from build123d import *

# Parameters (mm, degrees)
SKETCH1_W                 = 63.398443118
SKETCH1_H                 = 25.4
BOSS_EXTRUDE1_DEPTH       = 6.35
SKETCH2_W                 = 38.1
SKETCH2_H                 = 25.4
BOSS_EXTRUDE2_DEPTH       = 6.35
CUT_EXTRUDE3_DEPTH        = 60.875617776
TAP_DRILL_FOR_6_32_TAP1_D = 2.7051
F_1_4_CLEARANCE_HOLE1_D   = 6.7564


with BuildPart() as part:
    # Sketch1 → Boss-Extrude1 (new body)
    with BuildSketch(Plane.XY):
        with Locations((22.148778441, 406.4)):
            Rectangle(SKETCH1_W, SKETCH1_H)
    extrude(amount=BOSS_EXTRUDE1_DEPTH)

    # Sketch2 → Boss-Extrude2 (add)
    with BuildSketch(Plane(origin=(0, 0, 0), x_dir=(-1, 0, 0), z_dir=(0, 0, -1))):
        with Locations((-34.798, 406.4)):
            Rectangle(SKETCH2_W, SKETCH2_H)
    extrude(amount=BOSS_EXTRUDE2_DEPTH)

    # Sketch7 → Cut-Extrude3 (cut, through all)
    with BuildSketch(Plane(origin=(0, 419.1, 0), x_dir=(1, 0, 0), z_dir=(0, 1, 0))):
        with BuildLine():
            Line((-9.550443118, -0.242852773), (15.748, -0.242852773))
            ThreePointArc((15.748, -0.242852773), (15.919722843, -0.171722843), (15.990852773, 0))
            Line((15.990852773, 0), (15.990852773, 6.35))
            Line((15.990852773, 6.35), (15.748, 6.35))
            Line((15.748, 6.35), (15.748, 0))
            Line((15.748, 0), (-9.550443118, 0))
            Line((-9.550443118, 0), (-9.550443118, -0.242852773))
        make_face()
    extrude(amount=-CUT_EXTRUDE3_DEPTH, mode=Mode.SUBTRACT)

    # Tap Drill for #6-32 Tap1 (through all)
    with Locations(Plane.XY.offset(6.35)):
        with Locations((47.498, 406.4), (30.0355, 406.4)):
            Hole(TAP_DRILL_FOR_6_32_TAP1_D / 2)

    # 1/4 Clearance Hole1 (through all)
    with Locations(Plane.XY.offset(6.35)):
        with Locations((3.149556882, 406.4)):
            Hole(F_1_4_CLEARANCE_HOLE1_D / 2)


solid = part.part
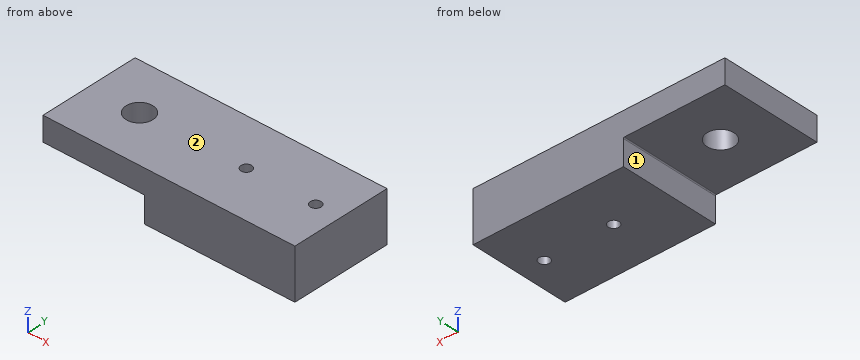
Can you work these out from the model? Positions are in its coordinate system, mm. Face numbers are marked on the shaded views. A direction names the side the tool comes from. Round coordinates to 2 decimals unless told otherwise and drop trailing zeros. Loops run counter-clockwise (first coordinate to the right, second up) from the corner with the lowest first, then second, coordinate; pieces in that order, holes last. Notation, with made-up numbers: (48, 54) - (98, 54) arc R33 ccw to (98, 88) - close; hole circle Ø3 at (74.5, 36). An arc over 180 degrees is marked (long way). Write item = value, one per line. Start each with the question number.
(1) If we section it at C-C (y = 413): Please give me the cut outline in (x, z).
(2) If I drill on probe 1 along X at (y, z) = (406.4, 2.75); probe 2 along X at (y, z) = (406.4, -0.75); probe 3 along Z at (x, y) = (-2.5, 395.75), over which ranges is the centre line in solid material (lowest first)? Write a range as [from, to].
(3) If we section it at A-A (z = 4.25): Please give me the cut outline in (x, y), and give its area (3 significant figures).
(4) For the marked faces 1 and 2, which set-ups out of +Z, -Z, +X, -X, +Y, -Y let a thin tool reach every point of the face, with its end or its side?
(5) For P1, Ø1.9, axis at y = 403.5, z = -1.5, coming from the -X side; P2, Ø12.5, axis at x = 7, y = 404.5, coming from the -Z side, each with a flat end and sliding along its axis, tell me the tip position at first contact or that it passes through.
(6) If we section it at B-B (y = 406.4): Please give me the cut outline in (x, z).
(7) If we section it at D-D (x = 1.5): Please give me the cut outline in (y, z).
Ans:
q1.outline = (-9.55, 0.24) - (15.75, 0.24) arc R0.24 cw to (15.99, 0) - (15.99, -6.35) - (53.85, -6.35) - (53.85, 6.35) - (-9.55, 6.35) - close
q2.probe_1 = [-9.55, -0.23], [6.53, 28.68], [31.39, 46.15], [48.85, 53.85]
q2.probe_2 = [15.99, 28.68], [31.39, 46.15], [48.85, 53.85]
q2.probe_3 = [0.24, 6.35]
q3.outline = (-9.55, 393.7) - (53.85, 393.7) - (53.85, 419.1) - (-9.55, 419.1) - close; hole circle Ø6.76 at (3.15, 406.4); hole circle Ø2.71 at (30.04, 406.4); hole circle Ø2.71 at (47.5, 406.4)
q3.area = 1,560 mm²
q4.face_1 = -Z, -X, +Y, -Y
q4.face_2 = +Z, +X, -X, +Y, -Y
q5.P1 = 15.99
q5.P2 = 0.24
q6.outline = (-9.55, 0.24) - (-0.23, 0.24) - (-0.23, 6.35) - (-9.55, 6.35) - close; (6.53, 0.24) - (15.75, 0.24) arc R0.24 cw to (15.99, 0) - (15.99, -6.35) - (28.68, -6.35) - (28.68, 6.35) - (6.53, 6.35) - close; (31.39, -6.35) - (46.15, -6.35) - (46.15, 6.35) - (31.39, 6.35) - close; (48.85, -6.35) - (53.85, -6.35) - (53.85, 6.35) - (48.85, 6.35) - close
q7.outline = (393.7, 0.24) - (403.45, 0.24) - (403.45, 6.35) - (393.7, 6.35) - close; (409.35, 0.24) - (419.1, 0.24) - (419.1, 6.35) - (409.35, 6.35) - close
